Work out the finished part from the listing and answer in its coordinate system (mm). A direction names the side the tool comes from. Coordinates: 2 decimals unless noted, no trailing zeros. Order: outer loops, then holes, each group sorted by start corner. A loop starts at its lowest first (then second) coordinate and runs counter-clockwise, first axis right, second up. Notation, with made-up numbers: M -17.75,10.25 L 39.25,10.25 A20 cw 39.25,41.25 Z; hole C 25.5,37.5 d11. An arc over 180 degrees is marked long. Use a Markdown table: item, result.
from build123d import *

# Parameters (mm, degrees)
F1_DEPTH = 5.842


with BuildPart() as f1:
    # F0 (on Front) → F1 (new body)
    with BuildSketch(Plane.XZ):
        with BuildLine():
            ThreePointArc((9.5433378796, -2.9874239932), (9.8851752336, -1.5110627392), (10, 0))
            ThreePointArc((10, 0), (9.8508269436, 1.7208162387), (9.4077582946, 3.3902925937))
            Line((9.4077582946, 3.3902925937), (5.7582254442, 0.1224102397))
            Line((5.7582254442, 0.1224102397), (9.5433378796, -2.9874239932))
        make_face()
        with BuildLine():
            ThreePointArc((9.4077582946, 3.3902925937), (9.8508269436, 1.7208162387), (10, 0))
            ThreePointArc((10, 0), (9.8851752336, -1.5110627392), (9.5433378796, -2.9874239932))
            Line((9.5433378796, -2.9874239932), (10.4715017977, -3.75))
            Line((10.4715017977, -3.75), (25, -3.75))
            Line((25, -3.75), (25, 3.75))
            Line((25, 3.75), (9.8094753252, 3.75))
            Line((9.8094753252, 3.75), (9.4077582946, 3.3902925937))
        make_face()
        with BuildLine():
            Line((5.7582254442, 0.1224102397), (9.4077582946, 3.3902925937))
            ThreePointArc((9.4077582946, 3.3902925937), (9.3407348831, 3.57080829), (9.2702481089, 3.75))
            Line((9.2702481089, 3.75), (3.43801843, 3.75))
            Line((3.43801843, 3.75), (3.43801843, 2.0286836526))
            Line((3.43801843, 2.0286836526), (5.7582254442, 0.1224102397))
        make_face()
        with BuildLine():
            ThreePointArc((9.2702481089, 3.75), (9.3407348831, 3.57080829), (9.4077582946, 3.3902925937))
            Line((9.4077582946, 3.3902925937), (9.8094753252, 3.75))
            Line((9.8094753252, 3.75), (9.2702481089, 3.75))
        make_face()
        with BuildLine():
            Line((10.4715017977, -3.75), (9.5433378796, -2.9874239932))
            ThreePointArc((9.5433378796, -2.9874239932), (9.4145172462, -3.3714781657), (9.2702481089, -3.75))
            Line((9.2702481089, -3.75), (10.4715017977, -3.75))
        make_face()
        with BuildLine():
            ThreePointArc((9.2702481089, -3.75), (9.4145172462, -3.3714781657), (9.5433378796, -2.9874239932))
            Line((9.5433378796, -2.9874239932), (5.7582254442, 0.1224102397))
            Line((5.7582254442, 0.1224102397), (3.43801843, -1.9551607454))
            Line((3.43801843, -1.9551607454), (3.43801843, -3.75))
            Line((3.43801843, -3.75), (9.2702481089, -3.75))
        make_face()
        with BuildLine():
            Line((3.43801843, 3.75), (9.2702481089, 3.75))
            ThreePointArc((9.2702481089, 3.75), (7.3200398798, 6.8130034609), (4.4046622613, 8.9776918172))
            Line((4.4046622613, 8.9776918172), (3.43801843, 8.1121349231))
            Line((3.43801843, 8.1121349231), (3.43801843, 3.75))
        make_face()
        with BuildLine():
            ThreePointArc((4.4046622613, 8.9776918172), (7.3200398798, 6.8130034609), (9.2702481089, 3.75))
            Line((9.2702481089, 3.75), (9.8094753252, 3.75))
            Line((9.8094753252, 3.75), (21.1996483638, 13.9490438251))
            Line((21.1996483638, 13.9490438251), (16.0986373051, 19.4487675029))
            Line((16.0986373051, 19.4487675029), (4.4046622613, 8.9776918172))
        make_face()
        Polygon((3.43801843, -1.9551607454), (5.7582254442, 0.1224102397), (3.43801843, 2.0286836526), align=None)
        with BuildLine():
            Line((10.4715017977, -3.75), (9.2702481089, -3.75))
            ThreePointArc((9.2702481089, -3.75), (7.4631867576, -6.6558878763), (4.7822119792, -8.7823942399))
            Line((4.7822119792, -8.7823942399), (16.6882236685, -18.5643289542))
            Line((16.6882236685, -18.5643289542), (21.7797240627, -13.0407931571))
            Line((21.7797240627, -13.0407931571), (10.4715017977, -3.75))
        make_face()
        with BuildLine():
            ThreePointArc((4.7822119792, -8.7823942399), (7.4631867576, -6.6558878763), (9.2702481089, -3.75))
            Line((9.2702481089, -3.75), (3.43801843, -3.75))
            Line((3.43801843, -3.75), (3.43801843, -7.6780098428))
            Line((3.43801843, -7.6780098428), (4.7822119792, -8.7823942399))
        make_face()
        with BuildLine():
            Line((3.43801843, 8.1121349231), (4.4046622613, 8.9776918172))
            ThreePointArc((4.4046622613, 8.9776918172), (3.926766698, 9.1967659152), (3.43801843, 9.3904222096))
            Line((3.43801843, 9.3904222096), (3.43801843, 8.1121349231))
        make_face()
        Polygon((1.3429305817, 3.75), (3.43801843, 3.75), (3.43801843, 8.1121349231), (-0.1050080786, 4.9396209927), align=None)
        Polygon((3.43801843, 2.0286836526), (3.43801843, 3.75), (1.3429305817, 3.75), align=None)
        Polygon((1.4335629107, -3.75), (3.43801843, -1.9551607454), (3.43801843, 2.0286836526), (1.3429305817, 3.75), (-1.4335629107, 3.75), (-4.06198157, 1.3964486531), (-4.06198157, -1.5160378684), (-1.3429305817, -3.75), align=None)
        with BuildLine():
            ThreePointArc((0, 1.6), (1.1313708499, 1.1313708499), (1.6, 0))
            ThreePointArc((1.6, 0), (1.1313708499, -1.1313708499), (0, -1.6))
            ThreePointArc((0, -1.6), (-1.6, 0), (0, 1.6))
        make_face(mode=Mode.SUBTRACT)
        Polygon((3.43801843, -3.75), (3.43801843, -1.9551607454), (1.4335629107, -3.75), align=None)
        with BuildLine():
            ThreePointArc((3.43801843, -9.3904222096), (4.1213434094, -9.1112308994), (4.7822119792, -8.7823942399))
            Line((4.7822119792, -8.7823942399), (3.43801843, -7.6780098428))
            Line((3.43801843, -7.6780098428), (3.43801843, -9.3904222096))
        make_face()
        Polygon((3.43801843, -7.6780098428), (3.43801843, -3.75), (1.4335629107, -3.75), (0.1050080786, -4.9396209927), align=None)
        with BuildLine():
            Line((3.43801843, 8.1121349231), (3.43801843, 9.3904222096))
            ThreePointArc((3.43801843, 9.3904222096), (-0.3365719222, 9.9943343621), (-4.06198157, 9.1378501698))
            Line((-4.06198157, 9.1378501698), (-4.06198157, 8.190655627))
            Line((-4.06198157, 8.190655627), (-0.1050080786, 4.9396209927))
            Line((-0.1050080786, 4.9396209927), (3.43801843, 8.1121349231))
        make_face()
        with BuildLine():
            ThreePointArc((-4.06198157, 9.1378501698), (-0.3365719222, 9.9943343621), (3.43801843, 9.3904222096))
            Line((3.43801843, 9.3904222096), (3.43801843, 24.7108984739))
            Line((3.43801843, 24.7108984739), (-4.06198157, 24.7108984739))
            Line((-4.06198157, 24.7108984739), (-4.06198157, 9.1378501698))
        make_face()
        Polygon((-1.4335629107, 3.75), (1.3429305817, 3.75), (-0.1050080786, 4.9396209927), align=None)
        Polygon((0.1050080786, -4.9396209927), (1.4335629107, -3.75), (-1.3429305817, -3.75), align=None)
        with BuildLine():
            Line((3.43801843, -25.2891015261), (3.43801843, -9.3904222096))
            ThreePointArc((3.43801843, -9.3904222096), (-0.3365719222, -9.9943343621), (-4.06198157, -9.1378501698))
            Line((-4.06198157, -9.1378501698), (-4.06198157, -25.2891015261))
            Line((-4.06198157, -25.2891015261), (3.43801843, -25.2891015261))
        make_face()
        with BuildLine():
            ThreePointArc((-4.06198157, -9.1378501698), (-0.3365719222, -9.9943343621), (3.43801843, -9.3904222096))
            Line((3.43801843, -9.3904222096), (3.43801843, -7.6780098428))
            Line((3.43801843, -7.6780098428), (0.1050080786, -4.9396209927))
            Line((0.1050080786, -4.9396209927), (-4.06198157, -8.6708470153))
            Line((-4.06198157, -8.6708470153), (-4.06198157, -9.1378501698))
        make_face()
        with BuildLine():
            Line((-4.06198157, 8.190655627), (-4.06198157, 9.1378501698))
            ThreePointArc((-4.06198157, 9.1378501698), (-4.4256668552, 8.9673559585), (-4.7822119792, 8.7823942399))
            Line((-4.7822119792, 8.7823942399), (-4.06198157, 8.190655627))
        make_face()
        Polygon((-1.4335629107, 3.75), (-0.1050080786, 4.9396209927), (-4.06198157, 8.190655627), (-4.06198157, 3.75), align=None)
        Polygon((-4.06198157, 1.3964486531), (-1.4335629107, 3.75), (-4.06198157, 3.75), align=None)
        Polygon((-4.06198157, -8.6708470153), (0.1050080786, -4.9396209927), (-1.3429305817, -3.75), (-4.06198157, -3.75), align=None)
        Polygon((-4.06198157, -3.75), (-1.3429305817, -3.75), (-4.06198157, -1.5160378684), align=None)
        with BuildLine():
            ThreePointArc((-4.4046622613, -8.9776918172), (-4.2340792524, -9.0593914191), (-4.06198157, -9.1378501698))
            Line((-4.06198157, -9.1378501698), (-4.06198157, -8.6708470153))
            Line((-4.06198157, -8.6708470153), (-4.4046622613, -8.9776918172))
        make_face()
        with BuildLine():
            Line((-4.06198157, 8.190655627), (-4.7822119792, 8.7823942399))
            ThreePointArc((-4.7822119792, 8.7823942399), (-7.4631867576, 6.6558878763), (-9.2702481089, 3.75))
            Line((-9.2702481089, 3.75), (-4.06198157, 3.75))
            Line((-4.06198157, 3.75), (-4.06198157, 8.190655627))
        make_face()
        with BuildLine():
            ThreePointArc((-9.2702481089, 3.75), (-7.4631867576, 6.6558878763), (-4.7822119792, 8.7823942399))
            Line((-4.7822119792, 8.7823942399), (-16.8534109154, 18.700046179))
            Line((-16.8534109154, 18.700046179), (-21.6145368158, 12.9050759323))
            Line((-21.6145368158, 12.9050759323), (-10.4715017977, 3.75))
            Line((-10.4715017977, 3.75), (-9.2702481089, 3.75))
        make_face()
        with BuildLine():
            Line((-5.7582254442, -0.1224102397), (-4.06198157, 1.3964486531))
            Line((-4.06198157, 1.3964486531), (-4.06198157, 3.75))
            Line((-4.06198157, 3.75), (-9.2702481089, 3.75))
            ThreePointArc((-9.2702481089, 3.75), (-9.4145172462, 3.3714781657), (-9.5433378796, 2.9874239932))
            Line((-9.5433378796, 2.9874239932), (-5.7582254442, -0.1224102397))
        make_face()
        Polygon((-4.06198157, -1.5160378684), (-4.06198157, 1.3964486531), (-5.7582254442, -0.1224102397), align=None)
        with BuildLine():
            Line((-4.4046622613, -8.9776918172), (-4.06198157, -8.6708470153))
            Line((-4.06198157, -8.6708470153), (-4.06198157, -3.75))
            Line((-4.06198157, -3.75), (-9.2702481089, -3.75))
            ThreePointArc((-9.2702481089, -3.75), (-7.3200398798, -6.8130034609), (-4.4046622613, -8.9776918172))
        make_face()
        with BuildLine():
            Line((-9.2702481089, -3.75), (-4.06198157, -3.75))
            Line((-4.06198157, -3.75), (-4.06198157, -1.5160378684))
            Line((-4.06198157, -1.5160378684), (-5.7582254442, -0.1224102397))
            Line((-5.7582254442, -0.1224102397), (-9.4077582946, -3.3902925937))
            ThreePointArc((-9.4077582946, -3.3902925937), (-9.3407348831, -3.57080829), (-9.2702481089, -3.75))
        make_face()
        with BuildLine():
            Line((-16.1475948178, -19.4926052757), (-4.4046622613, -8.9776918172))
            ThreePointArc((-4.4046622613, -8.9776918172), (-7.3200398798, -6.8130034609), (-9.2702481089, -3.75))
            Line((-9.2702481089, -3.75), (-9.8094753252, -3.75))
            Line((-9.8094753252, -3.75), (-21.1506908511, -13.9052060523))
            Line((-21.1506908511, -13.9052060523), (-16.1475948178, -19.4926052757))
        make_face()
        with BuildLine():
            ThreePointArc((-9.5433378796, 2.9874239932), (-9.4145172462, 3.3714781657), (-9.2702481089, 3.75))
            Line((-9.2702481089, 3.75), (-10.4715017977, 3.75))
            Line((-10.4715017977, 3.75), (-9.5433378796, 2.9874239932))
        make_face()
        with BuildLine():
            Line((-9.4077582946, -3.3902925937), (-5.7582254442, -0.1224102397))
            Line((-5.7582254442, -0.1224102397), (-9.5433378796, 2.9874239932))
            ThreePointArc((-9.5433378796, 2.9874239932), (-9.9977411832, -0.2125352519), (-9.4077582946, -3.3902925937))
        make_face()
        with BuildLine():
            Line((-9.8094753252, -3.75), (-9.2702481089, -3.75))
            ThreePointArc((-9.2702481089, -3.75), (-9.3407348831, -3.57080829), (-9.4077582946, -3.3902925937))
            Line((-9.4077582946, -3.3902925937), (-9.8094753252, -3.75))
        make_face()
        with BuildLine():
            ThreePointArc((-9.4077582946, -3.3902925937), (-9.9977411832, -0.2125352519), (-9.5433378796, 2.9874239932))
            Line((-9.5433378796, 2.9874239932), (-10.4715017977, 3.75))
            Line((-10.4715017977, 3.75), (-25, 3.75))
            Line((-25, 3.75), (-25, -3.75))
            Line((-25, -3.75), (-9.8094753252, -3.75))
            Line((-9.8094753252, -3.75), (-9.4077582946, -3.3902925937))
        make_face()
    extrude(amount=F1_DEPTH)


solid = f1.part
1. Section B-B on x = 17.5 is taken. Determine the outline of the cut face in (y, z), then the cut area to 3 significant figures.
Answers below:
| item | result |
|---|---|
| outline | M -5.84,-17.68 L 0,-17.68 L 0,-9.52 L -5.84,-9.52 Z; M -5.84,-3.75 L 0,-3.75 L 0,3.75 L -5.84,3.75 Z; M -5.84,10.64 L 0,10.64 L 0,17.94 L -5.84,17.94 Z |
| area | 134 mm² |
2. Section C-C on z = -15 is taken. Determine the outline of the cut face in (x, y).
Answers below:
| item | result |
|---|---|
| outline | M -20.17,-5.84 L -11.13,-5.84 L -11.13,0 L -20.17,0 Z; M -4.06,-5.84 L 3.44,-5.84 L 3.44,0 L -4.06,0 Z; M 12.35,-5.84 L 19.97,-5.84 L 19.97,0 L 12.35,0 Z |
3. Find the intervals of material crossed by probe 1 along Z at (x, y) = (-16.5, -2.35); probe 2 along Z at (x, y) = (-11.5, -3.85); probe 3 along X at (y, z) = (-0.95, 18), in increasing order.
Answers below:
| item | result |
|---|---|
| probe 1 | -19.1 to -9.74, -3.75 to 3.75, 8.7 to 18.41 |
| probe 2 | -15.33 to -5.26, -3.75 to 3.75, 4.6 to 14.3 |
| probe 3 | -17.43 to -16, -4.06 to 3.44, 14.48 to 17.44 |
4. Section D-D on z = -6 is taken. Determine the outline of the cut face in (x, y), then the cut area to 3 significant figures.
Answers below:
| item | result |
|---|---|
| outline | M -12.32,-5.84 L 13.21,-5.84 L 13.21,0 L -12.32,0 Z |
| area | 149 mm² |
5. Flat-ended cylindrical pins translate along their axes: P1, Ø1, axis at y = -4.5, z = -12, coming from the -X side; P2, Ø1.8, axis at x = 21, y = -2.5, coming from the +Z side; P3, Ø1.8, axis at x = -21, y = -4, coming from the -Z side. Find the tip coordinate at first contact, or state that the pin passes through.
Answers below:
| item | result |
|---|---|
| P1 | x = -19.58 |
| P2 | z = 15.13 |
| P3 | z = -15.08 |
6. For faces 1 (the face through (-10.73, -2.88, 13.67)), 2 (the face through (-18, -3, -3.75)), 3 (the face through (16.205, -2.88, -8.46)), 4 (the face through (3.438, -3, -17)), determine the directions among +Z, -Z, +X, -X, +Y, -Y from which every point of the face is accessible in a straight line to the end or side of a thin tool.
Answers below:
| item | result |
|---|---|
| face 1 | +Z, +Y, -Y |
| face 2 | -X, +Y, -Y |
| face 3 | +X, +Y, -Y |
| face 4 | -Z, +Y, -Y |
7. For a pull along Z with two mould halves and no side action, classify faces 5 (the face through (-25, -3, 0)), 6 (the face through (18, -3, -3.75)), 7 (the face through (0, -3, 24.711)) as +Z half, -Z half, draft (parallel to the pull), parting line (faces both ways), or undercut.
Answers below:
| item | result |
|---|---|
| face 5 | draft |
| face 6 | undercut |
| face 7 | +Z half |
